Read the model definition and answer for the solid it produces. Units are mm, in the model's axes. A direction names the side the tool comes from. Coordinates: 2 decimals unless noted, no trailing zeros. Write each loop counter-clockwise with the first axis right and the second up, starting at its lowest first coordinate (ties: lowest second). Pieces come first, ordered by that corner, then holes.
1) The part is cut by section B-B (z = 0). Determine the outline of the cut face in (x, y), then the cut area to 3 significant figures.
2) Find the intervals of material crossed by line 1 (Y direction, x = 161.5, z = 10.5); line 2 (X direction, y = 43, z = -1.5); line 3 (Z direction, x = -1, y = 78.5), in increasing order.
3) The part is cut by section A-A (x = 0). Determine the outline of the cut face in (y, z).
4) The part is cut by section D-D (y = 59.5). Determine the outline of the cut face in (x, z), then the cut area to 3 significant figures.
5) The part is cut by section C-C (y = -7). Determine the outline of the cut face in (x, z), then the cut area to 3 significant figures.
6) Which of the six approach directions +Z, -Z, +X, -X, +Y, -Y give full straight-line access (tool end or side, diameter ignored) to faces 1 (the face through (73, 0, -124)), 2 (the face through (-38.37, 41.06, 172.79))?
7) Each of these flat-tipped pins is pushed along its axis until it touches: pin 1 Ø2 at (x, y) = (-28, 58.5) entering from +Z; pin 2 Ø1.5 at (x, y) = (-114, 55.5) entering from +Z; pin 3 Ø1 at (x, y) = (22.5, 5) entering from -Z. Where does it stop, or does it pass through?
from build123d import *

# Parameters (mm, degrees)
SKETCH1_R           = 177
BOSS_EXTRUDE1_DEPTH = 83
FILLET1_R           = 10
SKETCH2_R           = 143.260231918
BOSS_EXTRUDE2_DEPTH = 15


with BuildPart() as part:
    # Sketch1 → Boss-Extrude1 (new body)
    with BuildSketch(Plane(origin=(0, 0, 0), x_dir=(1, 0, 0), z_dir=(0, 1, 0))):
        Circle(SKETCH1_R)
    extrude(amount=BOSS_EXTRUDE1_DEPTH)

    # Fillet1
    fillet1_edges = [part.edges().sort_by_distance(p)[0] for p in [
        (-177, 0, 0),
        (-177, 83, 0),
    ]]
    fillet(fillet1_edges, radius=FILLET1_R)

    # Sketch2 → Boss-Extrude2 (add)
    with BuildSketch(Plane.XZ):
        Circle(SKETCH2_R)
    extrude(amount=BOSS_EXTRUDE2_DEPTH)


solid = part.part
Reported:
1. outline: (-177, 10) arc R10 ccw to (-167, 0) - (-143.26, 0) - (-143.26, -15) - (143.26, -15) - (143.26, 0) - (167, 0) arc R10 ccw to (177, 10) - (177, 73) arc R10 ccw to (167, 83) - (-167, 83) arc R10 ccw to (-177, 73) - close
1. area: 33,600 mm2
2. line 1: y = 0 to 83
2. line 2: x = -176.99 to 176.99
2. line 3: z = -175.35 to 175.35
3. outline: (-15, -143.26) - (0, -143.26) - (0, -167) arc R10 ccw to (10, -177) - (73, -177) arc R10 ccw to (83, -167) - (83, 167) arc R10 ccw to (73, 177) - (10, 177) arc R10 ccw to (0, 167) - (0, 143.26) - (-15, 143.26) - close
4. outline: circle Ø354 at (0, 0)
4. area: 98,400 mm2
5. outline: circle Ø286.52 at (0, 0)
5. area: 64,500 mm2
6. face 1: -Y
6. face 2: +Y, -Y
7. pin 1: stops at z = 174.93
7. pin 2: stops at z = 136.03
7. pin 3: stops at z = -174.49
